The listing builds one solid part. Answer for the finished solid, in the listing's coordinates (mm). A direction names the side the tool comes from. Give positions to 0.01 mm unless a question says otherwise; leave off trailing zeros. Loops run counter-clockwise (first coordinate to the right, second up) from the corner with the lowest first, then second, coordinate; pieces in that order, holes last. Notation, with made-up numbers: (-22.5, -31.75) - (7.5, -31.75) arc R12 ccw to (7.5, -11.75) - close; hole circle Ø2 at (-5.5, -17.75). An arc over 180 degrees is marked (long way). Write item = value, one per line. Start each with the question number.
1) The part is cut by section C-C on y = -22.5. Write down the section's boundary in (x, z), plus the area to 3 significant figures.
2) Consider probe 1 along Y at (x, z) = (64.75, -150); probe 2 along X at (y, z) = (2.5, -84); probe 3 along Y at (x, z) = (23, -119.5). Determine where each line is inside the solid, lowest interval first.
3) Which of the six approach directions +Z, -Z, +X, -X, +Y, -Y give full straight-line access (tool end or side, diameter ignored) to faces 5 (the flat face through (35, 22, -120)), 6 (the flat face through (34.62, 23.35, -49.37)), 7 (the flat face through (66.198, -31.162, -76.05))?
4) The mould has two halves that part along Y. Classify faces 1 (the flat face through (3.698, -31.162, -76.05)), 2 (the cylindrical face through (66.198, 0.55, -174.994)), 3 (the flat face through (70, 1, -70)), 4 (the cylindrical face through (3.802, 0.33, 7.493)): +Y half, -Y half, draft (parallel to the pull), parting line (faces both ways), or undercut.
5) The part is cut by section D-D on z = -92. Write down the section's boundary in (x, y), plus the area to 3 significant figures.
6) Flat-ended cylindrical pins translate along their axes: P1, Ø5, axis at x = 34.5, z = -103.5, coming from the +Y side; P2, Ø11, axis at x = 47.5, y = 23.5, coming from the -Z side; P3, Ø8, axis at x = 57, z = -21, coming from the +Y side. Find the tip coordinate at first contact, or state that the pin passes through.
7) The part is cut by section B-B on z = -146. Write down the section's boundary in (x, y).
8) The part is cut by section A-A on y = 0. Write down the section's boundary in (x, z), plus the area to 3 significant figures.
from build123d import *

# Parameters (mm, degrees)
BOSS_EXTRUDE1_DEPTH     = 70
CUT_EXTRUDE1_DEPTH      = 193.17505041
CUT_EXTRUDE1_DEPTH_BACK = 193.17505041
SKETCH2_W               = 55
SKETCH2_H               = 55
CUT_EXTRUDE2_REACH      = 212.087
CUT_EXTRUDE2_START      = -10
SKETCH4_W               = 55
SKETCH4_H               = 159.369241685
SKETCH7_R               = 7.5
CUT_EXTRUDE4_DEPTH      = 193.17505041
SKETCH8_R               = 7.5
CUT_EXTRUDE5_DEPTH      = 193.17505041


with BuildPart() as part:
    # Sketch1 → Boss-Extrude1 (new body)
    with BuildSketch(Plane(origin=(0, 0, 0), x_dir=(0, 0, -1), z_dir=(1, 0, 0))):
        with BuildLine():
            Line((0, 37.5), (150, 25))
            ThreePointArc((150, 25), (175, 0), (150, -25))
            Line((150, -25), (0, -37.5))
            ThreePointArc((0, -37.5), (-37.5, 0), (0, 37.5))
        make_face()
    extrude(amount=BOSS_EXTRUDE1_DEPTH)

    # Sketch2 → Cut-Extrude1 (cut, two sides: drawn at the far end of the back side and taken through both)
    with BuildSketch(Plane(origin=(0, 0, 0), x_dir=(1, 0, 0), z_dir=(0, 1, 0)).offset(-CUT_EXTRUDE1_DEPTH_BACK)):
        with Locations((35, 147.5)):
            Rectangle(SKETCH2_W, SKETCH2_H)
    extrude(amount=CUT_EXTRUDE1_DEPTH + CUT_EXTRUDE1_DEPTH_BACK, mode=Mode.SUBTRACT)

    # Cut-Extrude2: up to this face of the body (flat: up to its plane)
    cut_extrude2_end = Plane(part.part.faces().sort_by_distance((35, -32.18220339, -63.813559322))[0])
    # Sketch4 → Cut-Extrude2 (cut, up to the picked face)
    with BuildSketch(Plane(origin=(0, 37.24137931, -3.103448276), x_dir=(1, 0, 0), z_dir=(0, 0.9965457582448797, -0.08304547985374003)).offset(CUT_EXTRUDE2_START), mode=Mode.PRIVATE) as cut_extrude2_sk1:
        with Locations((35, 42.184620843)):
            Rectangle(SKETCH4_W, SKETCH4_H)
    cut_extrude2_tool1 = split(extrude(cut_extrude2_sk1.sketch, amount=-CUT_EXTRUDE2_REACH, mode=Mode.PRIVATE), bisect_by=cut_extrude2_end, keep=Keep.BOTH, mode=Mode.PRIVATE)
    add(cut_extrude2_tool1.solids().sort_by(Axis((35, 23.77268, -44.311898), (0, -0.9965457582448797, 0.08304547985374003)))[0], mode=Mode.SUBTRACT)

    # Sketch7 → Cut-Extrude4 (cut, through all)
    with BuildSketch(Plane(origin=(70, 0, 0), x_dir=(0, 0, -1), z_dir=(1, 0, 0))):
        Circle(SKETCH7_R)
    extrude(amount=-CUT_EXTRUDE4_DEPTH, mode=Mode.SUBTRACT)

    # Sketch8 → Cut-Extrude5 (cut, through all)
    with BuildSketch(Plane(origin=(70, 0, 0), x_dir=(0, 0, -1), z_dir=(1, 0, 0))):
        with Locations((150, 0)):
            Circle(SKETCH8_R)
    extrude(amount=-CUT_EXTRUDE5_DEPTH, mode=Mode.SUBTRACT)


solid = part.part
Answer below:
q1.outline = (0, -160.9) - (7.5, -160.9) - (7.5, 30) - (0, 30) - close; (62.5, -160.9) - (70, -160.9) - (70, 30) - (62.5, 30) - close
q1.area = 2,860 mm2
q2.probe_1 = -25 to -7.5, 7.5 to 25
q2.probe_2 = 0 to 7.5, 62.5 to 70
q2.probe_3 = 17.51 to 27.54
q3.face_5 = -Z, +Y, -Y
q3.face_6 = +Z, -Y
q3.face_7 = -Z, +X, -X, -Y
q4.face_1 = -Y half
q4.face_2 = parting line
q4.face_3 = draft
q4.face_4 = undercut
q5.outline = (0, -29.83) - (7.5, -29.83) - (7.5, 19.8) - (62.5, 19.8) - (62.5, -29.83) - (70, -29.83) - (70, 29.83) - (0, 29.83) - close
q5.area = 1,450 mm2
q6.P1 = 29.08
q6.P2 = -120
q6.P3 = 36.08
q7.outline = (0, -25.33) - (7.5, -25.33) - (7.5, -6.34) - (0, -6.34) - close; (0, 6.34) - (7.5, 6.34) - (7.5, 25.33) - (0, 25.33) - close; (62.5, -25.33) - (70, -25.33) - (70, -6.34) - (62.5, -6.34) - close; (62.5, 6.34) - (70, 6.34) - (70, 25.33) - (62.5, 25.33) - close
q8.outline = (0, -175) - (7.5, -175) - (7.5, -157.5) - (0, -157.5) - close; (0, -142.5) - (7.5, -142.5) - (7.5, -7.5) - (0, -7.5) - close; (0, 7.5) - (7.5, 7.5) - (7.5, 37.5) - (0, 37.5) - close; (62.5, -175) - (70, -175) - (70, -157.5) - (62.5, -157.5) - close; (62.5, -142.5) - (70, -142.5) - (70, -7.5) - (62.5, -7.5) - close; (62.5, 7.5) - (70, 7.5) - (70, 37.5) - (62.5, 37.5) - close
q8.area = 2,740 mm2
